The listing builds one solid part. Answer for the finished solid, in the listing's coordinates (mm). Coordinates: 2 decimals unless noted, no trailing zeros. Loops run counter-clockwise (first coordinate to the right, second up) from the corner with the lowest first, then second, coordinate; pieces in that order, holes last. Notation, with made-up numbers: M 64.5,-26 L 107.5,-26 A29 cw 107.5,3 Z; hole C 23,-29 d11. An arc over 180 degrees is marked long. Answer as CSV lines item,"result". Start each with the question number.
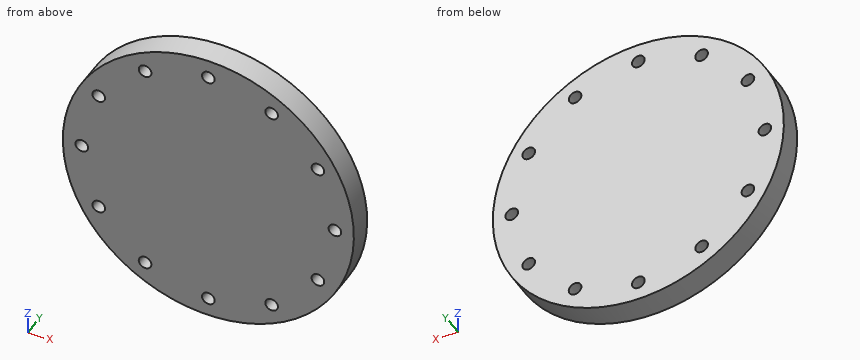
```python
from build123d import *

# Parameters (mm, degrees)
SKETCH1_R           = 115
BOSS_EXTRUDE1_DEPTH = 20
CUT_EXTRUDE1_REACH  = 165.86
SKETCH2_R           = 5


with BuildPart() as part:
    # Sketch1 → Boss-Extrude1 (new body)
    with BuildSketch(Plane(origin=(0, 0, 0), x_dir=(1, 0, 0), z_dir=(0, 1, 0))):
        with Locations(Location((0, 0, 0), (0, 0, 270))):
            Circle(SKETCH1_R)
    extrude(amount=BOSS_EXTRUDE1_DEPTH)

    # Sketch2 → Cut-Extrude1 (cut, up to next)
    with BuildSketch(Plane(origin=(0, 20, 0), x_dir=(1, 0, 0), z_dir=(0, 1, 0)), mode=Mode.PRIVATE) as cut_extrude1_sk1:
        with Locations(Location((0, 100, 0), (0, 0, 270))):
            Circle(SKETCH2_R)
    cut_extrude1_tool1 = extrude(cut_extrude1_sk1.sketch, amount=-CUT_EXTRUDE1_REACH, mode=Mode.PRIVATE) & part.part
    # Sketch2 → Cut-Extrude1 (cut, up to next)
    with BuildSketch(Plane(origin=(0, 20, 0), x_dir=(1, 0, 0), z_dir=(0, 1, 0)), mode=Mode.PRIVATE) as cut_extrude1_sk2:
        with Locations(Location((50, 86.602540378, 0), (0, 0, 270))):
            Circle(SKETCH2_R)
    cut_extrude1_tool2 = extrude(cut_extrude1_sk2.sketch, amount=-CUT_EXTRUDE1_REACH, mode=Mode.PRIVATE) & part.part
    # Sketch2 → Cut-Extrude1 (cut, up to next)
    with BuildSketch(Plane(origin=(0, 20, 0), x_dir=(1, 0, 0), z_dir=(0, 1, 0)), mode=Mode.PRIVATE) as cut_extrude1_sk3:
        with Locations(Location((86.602540378, 50, 0), (0, 0, 270))):
            Circle(SKETCH2_R)
    cut_extrude1_tool3 = extrude(cut_extrude1_sk3.sketch, amount=-CUT_EXTRUDE1_REACH, mode=Mode.PRIVATE) & part.part
    # Sketch2 → Cut-Extrude1 (cut, up to next)
    with BuildSketch(Plane(origin=(0, 20, 0), x_dir=(1, 0, 0), z_dir=(0, 1, 0)), mode=Mode.PRIVATE) as cut_extrude1_sk4:
        with Locations(Location((100, 0, 0), (0, 0, 270))):
            Circle(SKETCH2_R)
    cut_extrude1_tool4 = extrude(cut_extrude1_sk4.sketch, amount=-CUT_EXTRUDE1_REACH, mode=Mode.PRIVATE) & part.part
    # Sketch2 → Cut-Extrude1 (cut, up to next)
    with BuildSketch(Plane(origin=(0, 20, 0), x_dir=(1, 0, 0), z_dir=(0, 1, 0)), mode=Mode.PRIVATE) as cut_extrude1_sk5:
        with Locations(Location((86.602540378, -50, 0), (0, 0, 270))):
            Circle(SKETCH2_R)
    cut_extrude1_tool5 = extrude(cut_extrude1_sk5.sketch, amount=-CUT_EXTRUDE1_REACH, mode=Mode.PRIVATE) & part.part
    # Sketch2 → Cut-Extrude1 (cut, up to next)
    with BuildSketch(Plane(origin=(0, 20, 0), x_dir=(1, 0, 0), z_dir=(0, 1, 0)), mode=Mode.PRIVATE) as cut_extrude1_sk6:
        with Locations(Location((50, -86.602540378, 0), (0, 0, 270))):
            Circle(SKETCH2_R)
    cut_extrude1_tool6 = extrude(cut_extrude1_sk6.sketch, amount=-CUT_EXTRUDE1_REACH, mode=Mode.PRIVATE) & part.part
    # Sketch2 → Cut-Extrude1 (cut, up to next)
    with BuildSketch(Plane(origin=(0, 20, 0), x_dir=(1, 0, 0), z_dir=(0, 1, 0)), mode=Mode.PRIVATE) as cut_extrude1_sk7:
        with Locations(Location((0, -100, 0), (0, 0, 270))):
            Circle(SKETCH2_R)
    cut_extrude1_tool7 = extrude(cut_extrude1_sk7.sketch, amount=-CUT_EXTRUDE1_REACH, mode=Mode.PRIVATE) & part.part
    # Sketch2 → Cut-Extrude1 (cut, up to next)
    with BuildSketch(Plane(origin=(0, 20, 0), x_dir=(1, 0, 0), z_dir=(0, 1, 0)), mode=Mode.PRIVATE) as cut_extrude1_sk8:
        with Locations(Location((-50, -86.602540378, 0), (0, 0, 270))):
            Circle(SKETCH2_R)
    cut_extrude1_tool8 = extrude(cut_extrude1_sk8.sketch, amount=-CUT_EXTRUDE1_REACH, mode=Mode.PRIVATE) & part.part
    # Sketch2 → Cut-Extrude1 (cut, up to next)
    with BuildSketch(Plane(origin=(0, 20, 0), x_dir=(1, 0, 0), z_dir=(0, 1, 0)), mode=Mode.PRIVATE) as cut_extrude1_sk9:
        with Locations(Location((-86.602540378, -50, 0), (0, 0, 270))):
            Circle(SKETCH2_R)
    cut_extrude1_tool9 = extrude(cut_extrude1_sk9.sketch, amount=-CUT_EXTRUDE1_REACH, mode=Mode.PRIVATE) & part.part
    # Sketch2 → Cut-Extrude1 (cut, up to next)
    with BuildSketch(Plane(origin=(0, 20, 0), x_dir=(1, 0, 0), z_dir=(0, 1, 0)), mode=Mode.PRIVATE) as cut_extrude1_sk10:
        with Locations(Location((-100, 0, 0), (0, 0, 270))):
            Circle(SKETCH2_R)
    cut_extrude1_tool10 = extrude(cut_extrude1_sk10.sketch, amount=-CUT_EXTRUDE1_REACH, mode=Mode.PRIVATE) & part.part
    # Sketch2 → Cut-Extrude1 (cut, up to next)
    with BuildSketch(Plane(origin=(0, 20, 0), x_dir=(1, 0, 0), z_dir=(0, 1, 0)), mode=Mode.PRIVATE) as cut_extrude1_sk11:
        with Locations(Location((-86.602540378, 50, 0), (0, 0, 270))):
            Circle(SKETCH2_R)
    cut_extrude1_tool11 = extrude(cut_extrude1_sk11.sketch, amount=-CUT_EXTRUDE1_REACH, mode=Mode.PRIVATE) & part.part
    # Sketch2 → Cut-Extrude1 (cut, up to next)
    with BuildSketch(Plane(origin=(0, 20, 0), x_dir=(1, 0, 0), z_dir=(0, 1, 0)), mode=Mode.PRIVATE) as cut_extrude1_sk12:
        with Locations(Location((-50, 86.602540378, 0), (0, 0, 270))):
            Circle(SKETCH2_R)
    cut_extrude1_tool12 = extrude(cut_extrude1_sk12.sketch, amount=-CUT_EXTRUDE1_REACH, mode=Mode.PRIVATE) & part.part
    add(cut_extrude1_tool1.solids().sort_by_distance((0, 20, -100))[0], mode=Mode.SUBTRACT)
    add(cut_extrude1_tool2.solids().sort_by_distance((50, 20, -86.60254))[0], mode=Mode.SUBTRACT)
    add(cut_extrude1_tool3.solids().sort_by_distance((86.60254, 20, -50))[0], mode=Mode.SUBTRACT)
    add(cut_extrude1_tool4.solids().sort_by_distance((100, 20, 0))[0], mode=Mode.SUBTRACT)
    add(cut_extrude1_tool5.solids().sort_by_distance((86.60254, 20, 50))[0], mode=Mode.SUBTRACT)
    add(cut_extrude1_tool6.solids().sort_by_distance((50, 20, 86.60254))[0], mode=Mode.SUBTRACT)
    add(cut_extrude1_tool7.solids().sort_by_distance((0, 20, 100))[0], mode=Mode.SUBTRACT)
    add(cut_extrude1_tool8.solids().sort_by_distance((-50, 20, 86.60254))[0], mode=Mode.SUBTRACT)
    add(cut_extrude1_tool9.solids().sort_by_distance((-86.60254, 20, 50))[0], mode=Mode.SUBTRACT)
    add(cut_extrude1_tool10.solids().sort_by_distance((-100, 20, 0))[0], mode=Mode.SUBTRACT)
    add(cut_extrude1_tool11.solids().sort_by_distance((-86.60254, 20, -50))[0], mode=Mode.SUBTRACT)
    add(cut_extrude1_tool12.solids().sort_by_distance((-50, 20, -86.60254))[0], mode=Mode.SUBTRACT)


solid = part.part
```
Item 1: Consider line 1 (X direction, y = 6, z = 0); line 2 (Z direction, x = 52, y = 3.25); line 3 (X direction, y = 10.75, z = -50). Determine where each line is inside the solid, lowest interval first.
Item 2: Each of these flat-tipped pins is pushed along its axis until it touches: P1, Ø13, axis at x = -50, z = -86.6, coming from the +Y side; P2, Ø8, axis at x = 86.6, z = -50, coming from the -Y side; P3, Ø10, axis at x = -71, y = 14, coming from the +Z side; P4, Ø6, axis at x = -8, y = 10.5, coming from the +Z side. Where does it stop, or does it pass through?
Item 3: Section C-C on x = 100 is taken. Determine the outline of the cut face in (y, z), then the cut area to 3 significant figures.
Item 4: Section B-B on z = 0 is taken. Determine the outline of the cut face in (x, y).
Item 5: Section A-A on x = 0 is taken. Determine the outline of the cut face in (y, z).
Item 6: Section D-D on y = 13.5 is taken. State how many separate pieces and enclosed holes the cut face has, then the cut area to 3 significant figures.
Results are:
1,line 1,"-115 to -105, -95 to 95, 105 to 115"
1,line 2,"-102.57 to -91.19, -82.02 to 82.02, 91.19 to 102.57"
1,line 3,"-103.56 to -91.6, -81.6 to 81.6, 91.6 to 103.56"
2,P1,"y = 20"
2,P2,"through"
2,P3,"z = 94.18"
2,P4,"z = 114.89"
3,outline,"M 0,-56.79 L 20,-56.79 L 20,-5 L 0,-5 Z; M 0,5 L 20,5 L 20,56.79 L 0,56.79 Z"
3,area,"2,070 mm²"
4,outline,"M -115,0 L -105,0 L -105,20 L -115,20 Z; M -95,0 L 95,0 L 95,20 L -95,20 Z; M 105,0 L 115,0 L 115,20 L 105,20 Z"
5,outline,"M 0,-115 L 20,-115 L 20,-105 L 0,-105 Z; M 0,-95 L 20,-95 L 20,95 L 0,95 Z; M 0,105 L 20,105 L 20,115 L 0,115 Z"
6,separate pieces,"1"
6,enclosed holes,"12"
6,area,"40,600 mm²"
